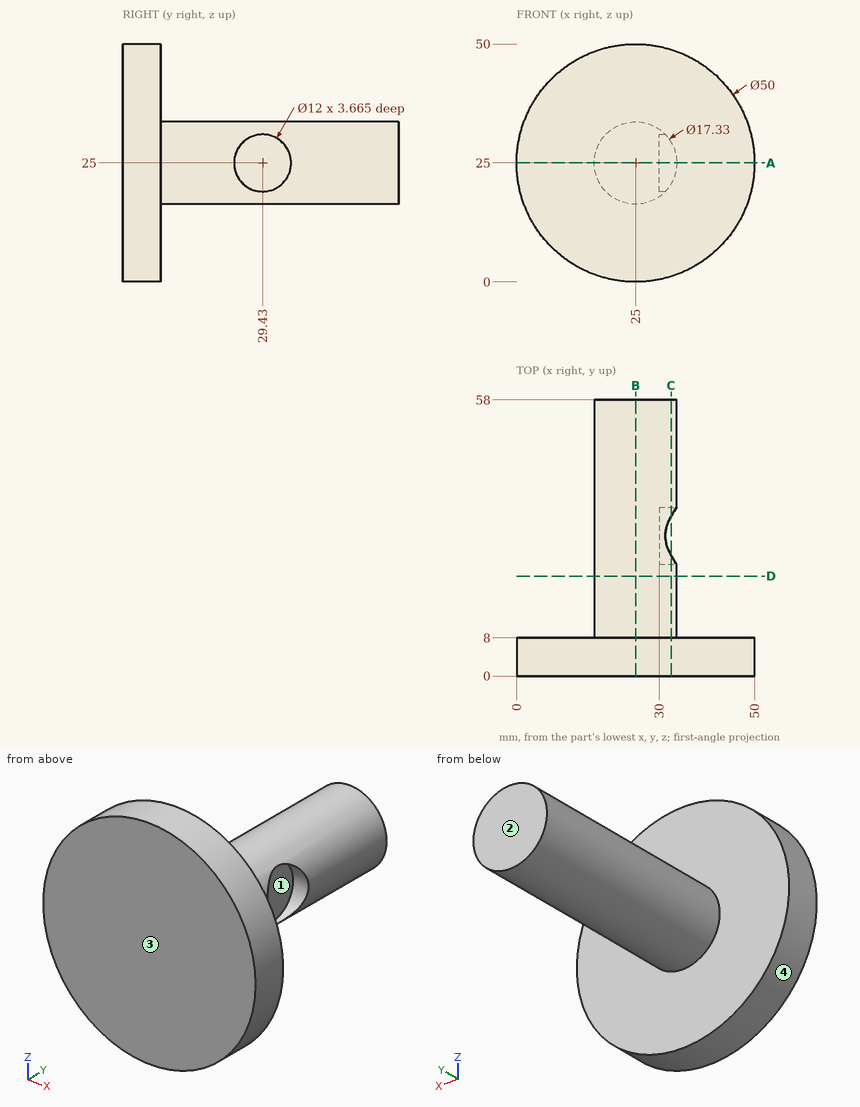
Print and shaded views of the part. All mm, measured from the part's lowest x, y and z. Give positions to 0.01 mm unless a question says otherwise; leave off trailing zeros. Loops run counter-clockwise (first coordinate to the right, second up) from the corner with the lowest first, then second, coordinate; pieces in that order, holes last. Notation, with made-up numbers: (55, -34.75) -> (73, -34.75) arc R4 cw to (73, -27.75) -> close; hole circle Ø7 at (84.25, -33). An arc over 180 degrees is marked (long way). Use a Markdown table: item, result.
1. Slice it at A-A (z = 25). List the corners of the cut face in (x, y) (3 decimals).
Check result:
| item | result |
|---|---|
| outline | (0, 0) -> (50, 0) -> (50, 8) -> (33.665, 8) -> (33.665, 23.43) -> (30, 23.43) -> (30, 35.43) -> (33.665, 35.43) -> (33.665, 58) -> (16.335, 58) -> (16.335, 8) -> (0, 8) -> close |
2. Flat gauge pins, fed straight in: pin 1 (10 mm diameter, centred on y = 38, z = 12, fed in from +X); pin 2 (4 mm diameter, centred on y = 49, z = 25.5, fed in from -X) (3 decimals); pin 3 (9.5 mm diameter, centred on y = 28.5, z = 24.5, fed in from +X). Where does each tip first touch, or does it go through?
Check result:
| item | result |
|---|---|
| pin 1 | stops at x = 28.33 |
| pin 2 | stops at x = 16.335 |
| pin 3 | stops at x = 30 |
3. Slice it at B-B (x = 25). List the corners of the cut face in (y, z) (3 decimals).
Check result:
| item | result |
|---|---|
| outline | (0, 0) -> (8, 0) -> (8, 16.335) -> (58, 16.335) -> (58, 33.665) -> (8, 33.665) -> (8, 50) -> (0, 50) -> close |
4. Mould opens along Y. For the marked faces 1, 2, 3 and 4 say: pulls with the +Y half, pulls with the -Y half, needs draft (parallel to the pull), parting line crosses it, or undercut.
Check result:
| item | result |
|---|---|
| face 1 | undercut |
| face 2 | pulls with the +Y half |
| face 3 | pulls with the -Y half |
| face 4 | needs draft |
5. Slice it at C-C (x = 32.5). List the corners of the cut face in (y, z).
Check result:
| item | result |
|---|---|
| outline | (0, 1.15) -> (8, 1.15) -> (8, 20.66) -> (25.29, 20.66) arc R6 cw to (25.29, 29.34) -> (8, 29.34) -> (8, 48.85) -> (0, 48.85) -> close; (33.57, 20.66) -> (58, 20.66) -> (58, 29.34) -> (33.57, 29.34) arc R6 cw to start |
6. Slice it at D-D (y = 21). List the corners of the cut face in (x, z) (3 decimals).
Check result:
| item | result |
|---|---|
| outline | circle Ø17.33 at (25, 25) |
7. Wall check: L1, parallel to Y at x = 32.15, z = 25; L2, parallel to X at y = 47, z = 25 (3 decimals); L3, parallel to Y at x = 35.5, z = 44.5. Give the ranges that are in metal, low to high. Write a range as [from, to].
Check result:
| item | result |
|---|---|
| L1 | y = [0, 23.43], [35.43, 58] |
| L2 | x = [16.335, 33.665] |
| L3 | y = [0, 8] |
